Geometry check sheet. Reference: drawing and pictorial views, mm from the part's lowest x, y, z. Give positions to 0.01 mm unless a question says otherwise; leave off trailing zeros. Loops run counter-clockwise (first coordinate to the right, second up) from the corner with the lowest first, then second, coordinate; pieces in that order, holes last. Notation, with made-up numbers: (45, 22) -> (66, 22) arc R26 cw to (66, 39) -> close; hole circle Ø8 at (73, -36). An arc over 180 degrees is marked (long way). Write each question's results on one line, items separated by ' | '. Start each with the question number.
1. Cross-section at B-B on x = 89.5. Record the boundary of the cut face in (y, z), and give its area (3 significant figures).
2. Gauge pin test, flat ends, axial feed: pin 1 Ø1.3 at (y, z) = (1, 104.5) entering from -X; pin 2 Ø1.4 at (x, y) = (12.5, 1.5) entering from +Z; pin 3 Ø1.3 at (y, z) = (1, 103.5) entering from +X. Record the tip position at first contact, or that the pin passes through.
3. Cross-section at A-A on y = 0.6. Record the boundary of the cut face in (x, z).
4. Material ranges on L1, parallel to Z at x = 123.5, y = 1.2, recorded low to high. Write a range as from..to.
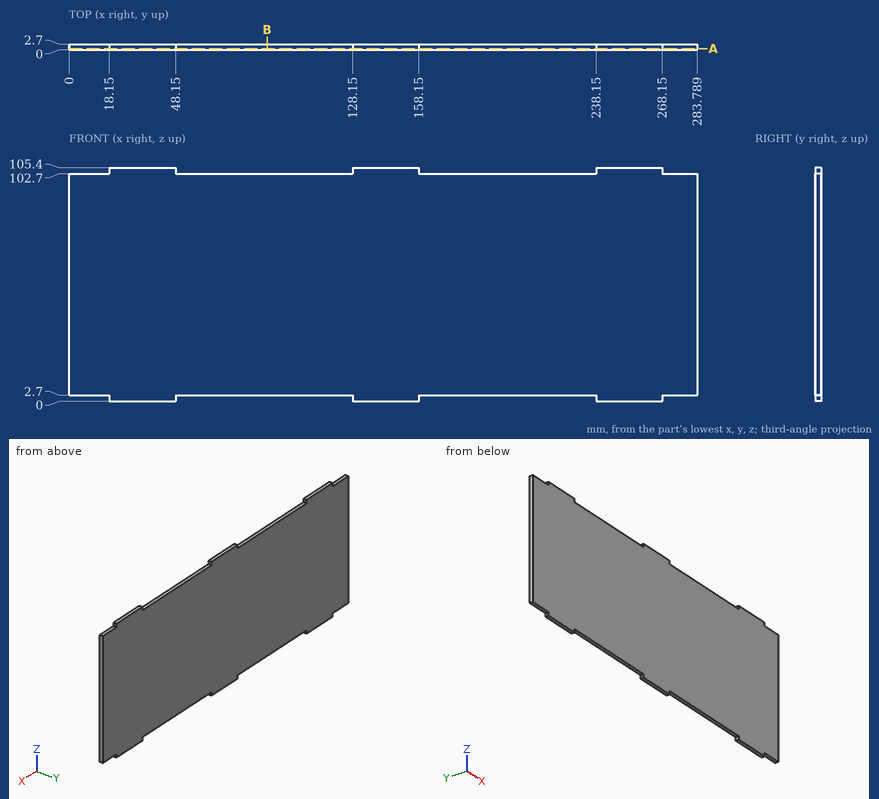
Geometry says:
1) outline: (0, 2.7) -> (2.7, 2.7) -> (2.7, 102.7) -> (0, 102.7) -> close | area: 270 mm^2
2) pin 1: x = 18.15 | pin 2: z = 102.7 | pin 3: x = 268.15
3) outline: (0, 2.7) -> (18.15, 2.7) -> (18.15, 0) -> (48.15, 0) -> (48.15, 2.7) -> (128.15, 2.7) -> (128.15, 0) -> (158.15, 0) -> (158.15, 2.7) -> (238.15, 2.7) -> (238.15, 0) -> (268.15, 0) -> (268.15, 2.7) -> (283.79, 2.7) -> (283.79, 102.7) -> (268.15, 102.7) -> (268.15, 105.4) -> (238.15, 105.4) -> (238.15, 102.7) -> (158.15, 102.7) -> (158.15, 105.4) -> (128.15, 105.4) -> (128.15, 102.7) -> (48.15, 102.7) -> (48.15, 105.4) -> (18.15, 105.4) -> (18.15, 102.7) -> (0, 102.7) -> close
4) L1: 2.7..102.7
